Could you check a few things on this model? Use its own coordinates, in mm. A direction names the side the tool comes from. Give positions to 0.01 mm unless a question says otherwise; leave off trailing zeros. Loops run counter-clockwise (first coordinate to the right, second up) from the corner with the lowest first, then second, coordinate; pieces in that order, holes last. Notation, with made-up numbers: (37.25, 85.25) -> (90.25, 85.25) arc R12 ccw to (90.25, 95.25) -> close; hole circle Ø11 at (47.5, 85). An arc over 180 degrees is marked (long way). Write each question's results on one line, items separated by ' | '. Start each with the question number.
Q1. If we section it at A-A, the plane z = 7.5: List the corners of the cut face in (x, y) for me, plus the area to 4 significant figures.
Q2. If we section it at B-B, the plane x = -19: List the corners of the cut face in (y, z) for me, plus the area to 3 significant figures.
Q3. If we section it at C-C, the plane y = -5.75: List the corners of the cut face in (x, z) for me, plus the area to 3 significant figures.
Q4. If we section it at D-D, the plane z = 1.5: List the corners of the cut face in (x, y) for me.
Q5. Which directions (+Z, -Z, +X, -X, +Y, -Y) give clear straight access to the entire face, cutting with the end or side of a thin tool? Please do faces 4 (the face through (-27.431, -3.5, 5.7)), 5 (the face through (-18, -9.636, 7)).
Q6. Will this pin go through, and if not, where does the flat tip stop? P1, Ø4, axis at y = -1, z = 8, coming from the +X side.
Q7. We'd pull the mould along Z, two halves only. Please class faces 1 (the face through (-23, -10, 15)), 2 (the face through (-25.931, -1, 7)), 3 (the face through (-26.7, -3.6, 9)): released by +Z, released by -Z, zero draft, split by the parting line, or undercut.
Q8. If I drill on line 1 along X through (y, z) = (-2, 2.5); line 2 along Y through (x, z) = (-27, 7.5); line 3 along Y through (x, z) = (-24.25, 11.5), over which ranges is the centre line in solid material (lowest first)?
from build123d import *

# Parameters (mm, degrees)
EXTRUSION1_DEPTH = 15
ESQUISSE2_R      = 1.5
EXTRUSION2_DEPTH = 15
ESQUISSE3_R      = 1.5
EXTRUSION3_DEPTH = 15


with BuildPart() as part:
    # Esquisse1 → Extrusion1 (new body)
    with BuildSketch(Plane.XY):
        Polygon((-27.431265327, 3.864105263), (-27.431265327, -11.135894737), (-12.431265327, -11.135894737), (-12.431265327, -9.635894737), (-25.931265327, -9.635894737), (-25.931265327, 3.864105263), align=None)
    extrude(amount=EXTRUSION1_DEPTH)

    # Esquisse2 → Extrusion2 (cut)
    with BuildSketch(Plane(origin=(-25.931265327, 0, 0), x_dir=(0, 0, -1), z_dir=(1, 0, 0))):
        with Locations((-7.5, -3.635894737)):
            Circle(ESQUISSE2_R)
    extrude(amount=-EXTRUSION2_DEPTH, mode=Mode.SUBTRACT)

    # Esquisse3 → Extrusion3 (cut)
    with BuildSketch(Plane(origin=(0, -9.635894737, 0), x_dir=(-1, 0, 0), z_dir=(0, 1, 0))):
        with Locations((19.931265327, 7.5)):
            Circle(ESQUISSE3_R)
    extrude(amount=-EXTRUSION3_DEPTH, mode=Mode.SUBTRACT)


solid = part.part
Final values:
1) outline: (-27.43, -11.14) -> (-21.43, -11.14) -> (-21.43, -9.64) -> (-25.93, -9.64) -> (-25.93, -5.14) -> (-27.43, -5.14) -> close; (-27.43, -2.14) -> (-25.93, -2.14) -> (-25.93, 3.86) -> (-27.43, 3.86) -> close; (-18.43, -11.14) -> (-12.43, -11.14) -> (-12.43, -9.64) -> (-18.43, -9.64) -> close | area: 33.75 mm²
2) outline: (-11.14, 0) -> (-9.64, 0) -> (-9.64, 6.32) -> (-11.14, 6.32) -> close; (-11.14, 8.68) -> (-9.64, 8.68) -> (-9.64, 15) -> (-11.14, 15) -> close | area: 19.0 mm²
3) outline: (-27.43, 0) -> (-25.93, 0) -> (-25.93, 15) -> (-27.43, 15) -> close | area: 22.5 mm²
4) outline: (-27.43, -11.14) -> (-12.43, -11.14) -> (-12.43, -9.64) -> (-25.93, -9.64) -> (-25.93, 3.86) -> (-27.43, 3.86) -> close
5) face 4: +Z, -Z, -X, +Y, -Y | face 5: +Z, -Z, +X, +Y
6) P1: stops at x = -25.93
7) face 1: released by +Z | face 2: zero draft | face 3: undercut
8) line 1: x = -27.43 to -25.93 | line 2: y = -11.14 to -5.14, -2.14 to 3.86 | line 3: y = -11.14 to -9.64
